```python
from build123d import *

# Parameters (mm, degrees)
F0_W     = 152.4
F0_H     = 152.4
F1_DEPTH = 152.4
F3_DEPTH = 152.4


with BuildPart() as f1:
    # F0 (on Top) → F1 (new body)
    with BuildSketch(Plane.XY):
        Rectangle(F0_W, F0_H)
    extrude(amount=F1_DEPTH)

    # F2 (on face) → F3 (cut)
    with BuildSketch(Plane.XY.offset(152.4)):
        Polygon((-25.422659, 44.033968), (-50.845865, 0.000315), (-25.423205, -44.033653), (25.422659, -44.033968), (50.845865, -0.000315), (25.423205, 44.033653), align=None)
    extrude(amount=-F3_DEPTH, mode=Mode.SUBTRACT)


solid = f1.part
```
The listing builds one solid part. Answer for the finished solid, in the listing's coordinates (mm). A direction names the side the tool comes from. Round coordinates to 2 decimals unless told otherwise and drop trailing zeros. Loops run counter-clockwise (first coordinate to the right, second up) from the corner with the lowest first, then second, coordinate; pieces in that order, holes last. Notation, with made-up numbers: (29, 53) - (63, 53) arc R13 cw to (63, 62) - close; hole circle Ø7 at (-16, 5). An arc over 180 degrees is marked (long way). Use one line per item in the form item = value. Start each with the question number.
1. The part is cut by section B-B on y = 38. Determine the outline of the cut face in (x, z).
2. A tool of negligible diameter and unlimited length cuts with its end or side. For faces 4 (the face through (37.956, -22.325, 77.267)), 5 (the face through (-1, 76.2, 75)), from which of +Z, -Z, +X, -X, +Y, -Y can it reach the whole face along a straight path? Write none if from no direction.
3. Consider line 1 (Y direction, x = -36, z = 78); line 2 (Y direction, x = 7.5, z = 19.5); line 3 (X direction, y = 3, z = 79.5). Determine where each line is inside the solid, lowest interval first. Write a range as [from, to].
4. The part is cut by section C-C on z = 138.5. Determine the outline of the cut face in (x, y).
5. Given pin 1 Ø3 at (x, y) = (8.5, -55) entering from -Z, flat-ended and moving along its own axis, determine where the tip first touches the part or whether it passes through.
6. The part is cut by section A-A on x = 32. Determine the outline of the cut face in (y, z).
7. For a pull along X with two mould halves and no side action, classify faces 1 (the face through (-35, 35, 0)), 2 (the face through (76.2, -1, 75)), 3 (the face through (-37.956, 22.325, 77.267)) as pulls with the +X half, pulls with the -X half, needs draft (parallel to the pull), parting line crosses it, or undercut.
Geometry check:
q1.outline = (-76.2, 0) - (-28.91, 0) - (-28.91, 152.4) - (-76.2, 152.4) - close; (28.91, 0) - (76.2, 0) - (76.2, 152.4) - (28.91, 152.4) - close
q2.face_4 = +Z, -Z
q2.face_5 = +Z, -Z, +X, -X, +Y
q3.line_1 = [-76.2, -25.71], [25.71, 76.2]
q3.line_2 = [-76.2, -44.03], [44.03, 76.2]
q3.line_3 = [-76.2, -49.11], [49.11, 76.2]
q4.outline = (-76.2, -76.2) - (76.2, -76.2) - (76.2, 76.2) - (-76.2, 76.2) - close; hole (-50.85, 0) - (-25.42, -44.03) - (25.42, -44.03) - (50.85, 0) - (25.42, 44.03) - (-25.42, 44.03) - close
q5.pin_1 = 0
q6.outline = (-76.2, 0) - (-32.64, 0) - (-32.64, 152.4) - (-76.2, 152.4) - close; (32.64, 0) - (76.2, 0) - (76.2, 152.4) - (32.64, 152.4) - close
q7.face_1 = needs draft
q7.face_2 = pulls with the +X half
q7.face_3 = undercut
